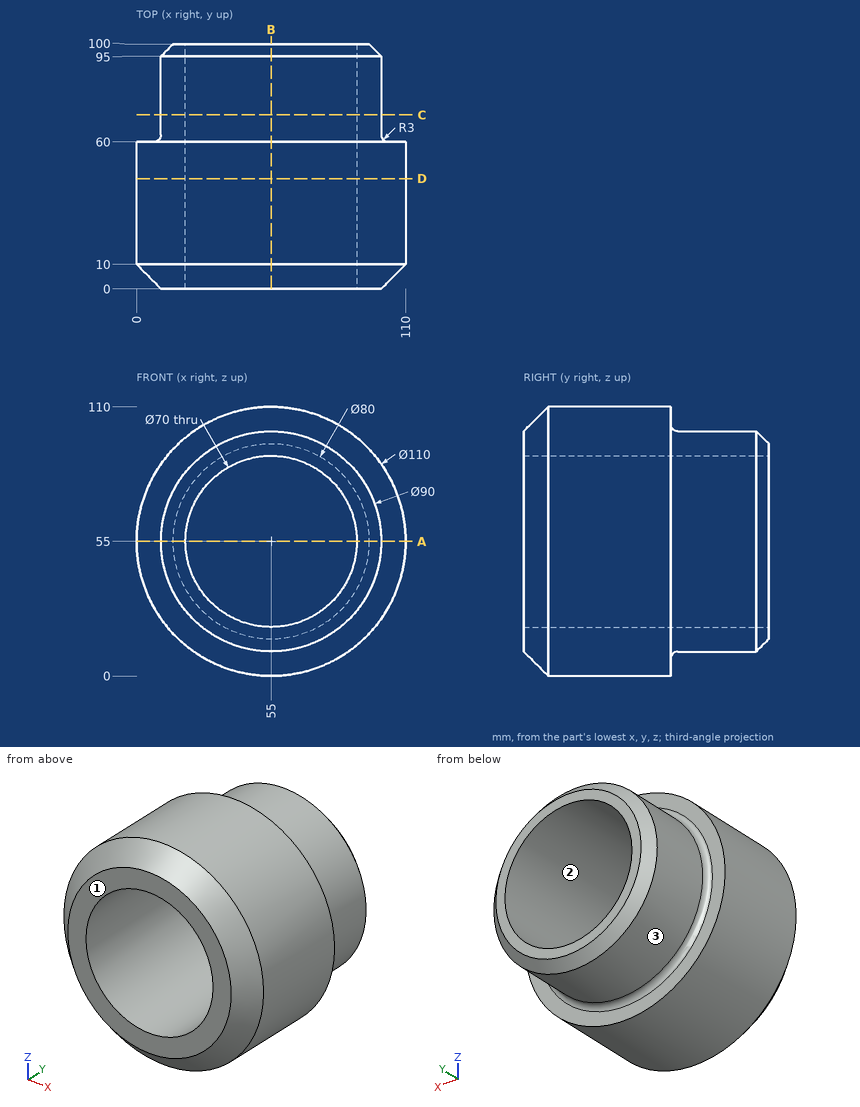
Job drawing, mm, ordinate dimensions from the low corner. One solid piece. Round coordinates to 2 decimals unless told otherwise and drop trailing zeros. Loops run counter-clockwise (first coordinate to the right, second up) from the corner with the lowest first, then second, coordinate; pieces in that order, holes last.
(1) Wall check: line 1 along X through (y, z) = (43, 55); line 2 along X through (y, z) = (63, 55). Give the ranges that are in metal, low to high.
(2) Cut at C-C (y = 71). Give the cut face in (x, z).
(3) Cut at D-D (y = 45). Give the cut face in (x, z).
(4) Drop flat-ended pins along their axis: pin 1 (1 mm diameter, centred on x = 68, y = 85, fed in from +Z); pin 2 (1 mm diameter, centred on y = 59, z = 75.5, fed in from -X); pin 3 (10 mm diameter, centred on y = 82.5, z = 58, fed in from -X). Give the stop position or say it passes through.
(5) Cut at B-B (x = 55). Give the cut face in (y, z), plus the area to 3 significant figures.
(6) Two-plate mould, pull along X, no slides. Class the marked faces 1, 2 and 3: +X half, -X half, draft (parallel to the pull), parting line (faces both ways), or undercut.
(7) Cut at A-A (z = 55). Give the cut face in (x, y), plus the area to 3 significant figures.
Findings below:
1. line 1: x = 0 to 20, 90 to 110
1. line 2: x = 10 to 20, 90 to 100
2. outline: circle Ø90 at (55, 55); hole circle Ø70 at (55, 55)
3. outline: circle Ø110 at (55, 55); hole circle Ø70 at (55, 55)
4. pin 1: stops at z = 98.23
4. pin 2: stops at x = 3.77
4. pin 3: stops at x = 10
5. outline: (0, 10) - (10, 0) - (60, 0) - (60, 7) arc R3 cw to (63, 10) - (95, 10) - (100, 15) - (100, 20) - (0, 20) - close; (0, 90) - (100, 90) - (100, 95) - (95, 100) - (63, 100) arc R3 cw to (60, 103) - (60, 110) - (10, 110) - (0, 100) - close
5. area: 3,080 mm2
6. face 1: draft
6. face 2: undercut
6. face 3: parting line
7. outline: (0, 10) - (10, 0) - (20, 0) - (20, 100) - (15, 100) - (10, 95) - (10, 63) arc R3 cw to (7, 60) - (0, 60) - close; (90, 0) - (100, 0) - (110, 10) - (110, 60) - (103, 60) arc R3 cw to (100, 63) - (100, 95) - (95, 100) - (90, 100) - close
7. area: 3,080 mm2
